from build123d import *

# Parameters (mm, degrees)
SKETCH1_W           = 358.775
SKETCH1_H           = 358.775
BOSS_EXTRUDE1_DEPTH = 3.175
SKETCH2_R           = 4.7625
CUT_EXTRUDE1_DEPTH  = 4.175


with BuildPart() as part:
    # Sketch1 → Boss-Extrude1 (new body)
    with BuildSketch(Plane(origin=(0, 0, 0), x_dir=(1, 0, 0), z_dir=(0, 1, 0))):
        with Locations((179.3875, 179.3875)):
            Rectangle(SKETCH1_W, SKETCH1_H)
    extrude(amount=BOSS_EXTRUDE1_DEPTH)

    # Sketch2 → Cut-Extrude1 (cut, through all)
    with BuildSketch(Plane(origin=(0, 3.175, 0), x_dir=(1, 0, 0), z_dir=(0, 1, 0))):
        with Locations((44.45, 12.7)):
            Circle(SKETCH2_R)
        with Locations((69.85, 12.7)):
            Circle(SKETCH2_R)
        with Locations((317.5, 12.7)):
            Circle(SKETCH2_R)
        with Locations((342.9, 12.7)):
            Circle(SKETCH2_R)
    cut_extrude1 = extrude(amount=-CUT_EXTRUDE1_DEPTH, mode=Mode.SUBTRACT)

    # Mirror1: Cut-Extrude1 across plane
    add(cut_extrude1.mirror(Plane.XY.offset(-179.3875)), mode=Mode.SUBTRACT)


solid = part.part
Geometry check sheet. Reference: the model listing, model coordinates, mm. Round coordinates to 2 decimals unless told otherwise and drop trailing zeros. Write each loop counter-clockwise with the first axis right and the second up, starting at its lowest first coordinate (ties: lowest second). Pieces come first, ordered by that corner, then holes. Notation, with made-up numbers: (88.5, 28) - (92.5, 28) arc R14 ccw to (92.5, 52) - close; hole circle Ø9 at (77, 0.25). An arc over 180 degrees is marked (long way). One line per item, written item: value.
1. Cross-section at A-A on x = 44.45. Record the boundary of the cut face in (y, z) (1 decimal).
The answers:
outline: (0, -358.8) - (3.2, -358.8) - (3.2, -350.8) - (0, -350.8) - close; (0, -341.3) - (3.2, -341.3) - (3.2, -17.5) - (0, -17.5) - close; (0, -7.9) - (3.2, -7.9) - (3.2, 0) - (0, 0) - close
2. Cross-section at B-B on z = -12.7. Record the boundary of the cut face in (x, y) (1 decimal), and give its area (3 significant figures).
The answers:
outline: (0, 0) - (39.7, 0) - (39.7, 3.2) - (0, 3.2) - close; (49.2, 0) - (65.1, 0) - (65.1, 3.2) - (49.2, 3.2) - close; (74.6, 0) - (312.7, 0) - (312.7, 3.2) - (74.6, 3.2) - close; (322.3, 0) - (338.1, 0) - (338.1, 3.2) - (322.3, 3.2) - close; (347.7, 0) - (358.8, 0) - (358.8, 3.2) - (347.7, 3.2) - close
area: 1,020 mm^2
3. Scan lines: L1, parallel to Z at x = 44.45, y = 1.75 (1 decimal); L2, parallel to X at y = 0.85, z = -12.7 (1 decimal); L3, parallel to Z at x = 313.5, y = 1.85 (3 decimals). Record each from-to range of solid material in increasing order.
The answers:
L1: z = -358.8 to -350.8, -341.3 to -17.5, -7.9 to 0
L2: x = 0 to 39.7, 49.2 to 65.1, 74.6 to 312.7, 322.3 to 338.1, 347.7 to 358.8
L3: z = -358.775 to -348.66, -343.49 to -15.285, -10.115 to 0
4. Mould release check, pull along X, two halves, no side actions. Record for faces 1 (the face through (347.44, 1.61, -344.64)), 2 (the face through (177, 0, -182)): released by +X, released by -X, zero draft, split by the parting line, or undercut.
The answers:
face 1: undercut
face 2: zero draft
